The listing builds one solid part. Answer for the finished solid, in the listing's coordinates (mm). A direction names the side the tool comes from. Coordinates: 2 decimals unless noted, no trailing zeros. Loops run counter-clockwise (first coordinate to the right, second up) from the corner with the lowest first, then second, coordinate; pieces in that order, holes last. Notation, with made-up numbers: (39.5, -11.5) - (77.5, -11.5) arc R17 cw to (77.5, 15.5) - close; hole circle Ø6 at (39.25, 71). An arc over 180 degrees is marked (long way). One line per question, with ' | ' between items.
from build123d import *

# Parameters (mm, degrees)
SKETCH1_W           = 10
SKETCH1_H           = 13
SKETCH1_R           = 1.65
BOSS_EXTRUDE1_DEPTH = 6
CUT_EXTRUDE1_DEPTH  = 2.4
SKETCH3_W           = 10
SKETCH3_H           = 58
BOSS_EXTRUDE2_DEPTH = 3
SKETCH4_R           = 1.65
CUT_EXTRUDE2_DEPTH  = 3


with BuildPart() as part:
    # Sketch1 → Boss-Extrude1 (new body)
    with BuildSketch(Plane(origin=(0, 0, 0), x_dir=(1, 0, 0), z_dir=(0, 1, 0))):
        with Locations((0, 1.5)):
            Rectangle(SKETCH1_W, SKETCH1_H)
        Circle(SKETCH1_R, mode=Mode.SUBTRACT)
    extrude(amount=BOSS_EXTRUDE1_DEPTH)

    # Sketch2 → Cut-Extrude1 (cut)
    with BuildSketch(Plane(origin=(0, 6, 0), x_dir=(1, 0, 0), z_dir=(0, 1, 0))):
        Polygon((3.175426481, 0), (1.58771324, 2.75), (-1.58771324, 2.75), (-3.175426481, 0), (-1.58771324, -2.75), (1.58771324, -2.75), align=None)
    extrude(amount=-CUT_EXTRUDE1_DEPTH, mode=Mode.SUBTRACT)

    # Sketch3 → Boss-Extrude2 (add)
    with BuildSketch(Plane(origin=(0, 0, -8), x_dir=(-1, 0, 0), z_dir=(0, 0, -1))):
        with Locations((0, 29)):
            Rectangle(SKETCH3_W, SKETCH3_H)
    extrude(amount=-BOSS_EXTRUDE2_DEPTH)

    # Sketch4 → Cut-Extrude2 (cut)
    with BuildSketch(Plane.XY.offset(-5)):
        with Locations((0, 50)):
            Circle(SKETCH4_R)
    extrude(amount=-CUT_EXTRUDE2_DEPTH, mode=Mode.SUBTRACT)


solid = part.part
Item 1: Find section C-C, the plane z = -0.5. Write down the section's boundary in (x, y), plus the area to 3 significant figures.
Taken from the geometry:
outline: (-5, 0) - (-1.57, 0) - (-1.57, 3.6) - (-2.89, 3.6) - (-2.89, 6) - (-5, 6) - close; (1.57, 0) - (5, 0) - (5, 6) - (2.89, 6) - (2.89, 3.6) - (1.57, 3.6) - close | area: 34.8 mm2
Item 2: Find section B-B, the plane y = 50. Write down the section's boundary in (x, z), plus the area to 3 significant figures.
Taken from the geometry:
outline: (-5, -8) - (-1.65, -8) - (-1.65, -5) - (-5, -5) - close; (1.65, -8) - (5, -8) - (5, -5) - (1.65, -5) - close | area: 20.1 mm2
Item 3: Find section D-D, the plane x = -3.75. Write down the section's boundary in (y, z).
Taken from the geometry:
outline: (0, -8) - (58, -8) - (58, -5) - (6, -5) - (6, 5) - (0, 5) - close
Item 4: Which of the six approach directions +Z, -Z, +X, -X, +Y, -Y give full straight-line access (tool end or side, diameter ignored) to faces 5 (the face through (-2.37, 4.817, -1.394)), 6 (the face through (-1.216, 1.775, -1.115)), 7 (the face through (2.2, 6, -2.3))?
Taken from the geometry:
face 5: +Y | face 6: +Y, -Y | face 7: +Z, +X, -X, +Y
Item 5: Each of these flat-tipped pins is pushed along its axis until it touches: pin 1 Ø3 at (x, z) = (0, -0.5) entering from +Y; pin 2 Ø2 at (x, z) = (-2, -1) entering from +Y; pin 3 Ø4 at (x, y) = (2, 42) entering from +Z. Where does it stop, or does it pass through?
Taken from the geometry:
pin 1: stops at y = 3.6 | pin 2: stops at y = 6 | pin 3: stops at z = -5
Item 6: Find the intervals of material crossed by line 1 (Y direction, x = 0, z = -6.2); line 2 (Z direction, x = 0, y = 2.1); line 3 (X direction, y = 1.45, z = 0), in increasing order. Write a range as [from, to].
Taken from the geometry:
line 1: y = [0, 48.35], [51.65, 58] | line 2: z = [-8, -1.65], [1.65, 5] | line 3: x = [-5, -1.65], [1.65, 5]
Item 7: Find section A-A, the plane x = 0. Write down the section's boundary in (y, z).
Taken from the geometry:
outline: (0, -8) - (48.35, -8) - (48.35, -5) - (6, -5) - (6, -2.75) - (3.6, -2.75) - (3.6, -1.65) - (0, -1.65) - close; (0, 1.65) - (3.6, 1.65) - (3.6, 2.75) - (6, 2.75) - (6, 5) - (0, 5) - close; (51.65, -8) - (58, -8) - (58, -5) - (51.65, -5) - close
Item 8: The mould has two halves that part along Z. Classify faces 1 (the face through (0, 29, -8)), 2 (the face through (0, 3, 5)), 3 (the face through (0.89, 51.39, -6.48)), 4 (the face through (2.37, 4.817, 1.394)): pulls with the +Z half, pulls with the -Z half, needs draft (parallel to the pull), parting line crosses it, or undercut.
Taken from the geometry:
face 1: pulls with the -Z half | face 2: pulls with the +Z half | face 3: needs draft | face 4: undercut
